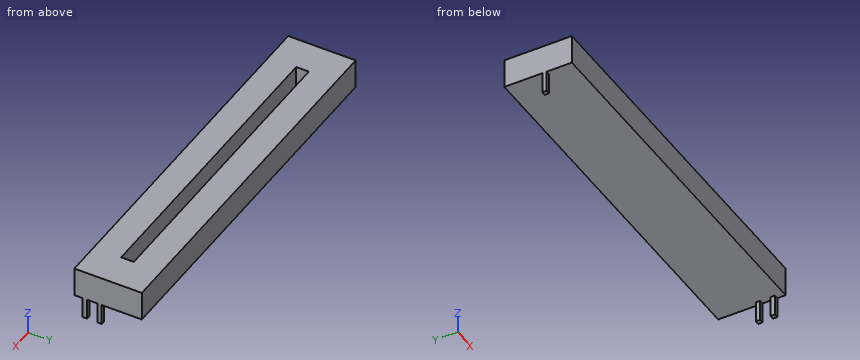
```python
from build123d import *

# Parameters (mm, degrees)
F0_W     = 88
F0_H     = 16
F1_DEPTH = 7
F2_W     = 72
F2_H     = 3
F3_DEPTH = 5
F4_W     = 1
F4_H     = 1
F5_DEPTH = 5


with BuildPart() as f1:
    # F0 (on Top) → F1 (new body)
    with BuildSketch(Plane.XY):
        Rectangle(F0_W, F0_H)
    extrude(amount=F1_DEPTH)

    # F2 (on face) → F3 (cut)
    with BuildSketch(Plane.XY.offset(7)):
        Rectangle(F2_W, F2_H)
    extrude(amount=-F3_DEPTH, mode=Mode.SUBTRACT)

    # F4 (on face) → F5 (join)
    with BuildSketch(Plane(origin=(0, 0, 0), x_dir=(1, 0, 0), z_dir=(0, 0, -1))):
        with Locations((-43.5, 1.5)):
            Rectangle(F4_W, F4_H)
        with Locations((43.5, 5.5)):
            Rectangle(F4_W, F4_H)
        with Locations((43.5, 2)):
            Rectangle(F4_W, F4_H)
    extrude(amount=F5_DEPTH)


solid = f1.part
```
Model file for the job. Use its own axes, mm. Coordinates: 2 decimals unless noted, no trailing zeros. Loops run counter-clockwise (first coordinate to the right, second up) from the corner with the lowest first, then second, coordinate; pieces in that order, holes last. Notation, with made-up numbers: (21, 52.25) - (67, 52.25) arc R19 ccw to (67, 68.25) - close; hole circle Ø5 at (47.5, -29.75). An arc over 180 degrees is marked (long way). Answer as a JSON object with one key per item and string values. Group by question number.
(1) Cut at B-B (x = -34). Give the cut face in (y, z), then the cut area to 3 significant figures.
(2) Flat gauge pins, fed straight in: pin 1 (2 mm diameter, centred on x = 14, y = 1, fed in from -Z); pin 2 (0.9 mm diameter, centred on x = -14, y = 0, fed in from +Z); pin 3 (1.1 mm diameter, centred on x = 43.5, z = -2, fed in from +Y). Where does each tip first touch, or does it go through?
(3) Probe line 1 along Y through (x, z) = (35, 4); line 2 along X through (y, z) = (1, 5.5); line 3 along Z through (x, y) = (2.5, -6.5). List the from-to ranges inside material, lowest first.
(4) Cut at D-D (x = 39). Give the cut face in (y, z).
(5) Cut at C-C (y = 0.5). Give the cut face in (x, z), then the cut area to 3 significant figures.
(6) Cut at A-A (z = -3.5). Give the cut face in (x, y), then the cut area to 3 significant figures.
Geometry says:
{
 "1": {"outline": "(-8, 0) - (8, 0) - (8, 7) - (1.5, 7) - (1.5, 2) - (-1.5, 2) - (-1.5, 7) - (-8, 7) - close", "area": "97.0 mm^2"},
 "2": {"pin 1": "stops at z = 0", "pin 2": "stops at z = 2", "pin 3": "stops at y = -1.5"},
 "3": {"line 1": "y = -8 to -1.5, 1.5 to 8", "line 2": "x = -44 to -36, 36 to 44", "line 3": "z = 0 to 7"},
 "4": {"outline": "(-8, 0) - (8, 0) - (8, 7) - (-8, 7) - close"},
 "5": {"outline": "(-44, 0) - (44, 0) - (44, 7) - (36, 7) - (36, 2) - (-36, 2) - (-36, 7) - (-44, 7) - close", "area": "256 mm^2"},
 "6": {"outline": "(-44, -2) - (-43, -2) - (-43, -1) - (-44, -1) - close; (43, -6) - (44, -6) - (44, -5) - (43, -5) - close; (43, -2.5) - (44, -2.5) - (44, -1.5) - (43, -1.5) - close", "area": "3.00 mm^2"}
}
